Input: part model. Units: mm. Frame: model coordinates. Face numbers are marked on the shaded views. A direction names the side the tool comes from. Round coordinates to 2 decimals unless told otherwise and drop trailing zeros. Order: outer loops, then holes, each group sorted by start corner. A loop starts at its lowest first (then second) coordinate and runs counter-clockwise, first axis right, second up. Notation, with made-up numbers: (-9.75, 15.25) - (26.25, 15.25) arc R32 ccw to (26.25, 48.25) - close; hole circle Ø8 at (26, 26.25). An arc over 180 degrees is marked (long way). One line per item, written item: value. Start each with the question number.
Autodesk Inventor part; units mm, degrees
ref_plane "WorkPlane2" through (0, 0, 0) normal (0, 0, 1) x (1, 0, 0)
ref_plane "Work Plane2" through (0, 0, -2.35) normal (0, 0, 1) x (1, 0, 0)
ref_plane "WorkPlane3" through (0, 0, 7) normal (0, 0, 1) x (1, 0, 0)
ref_plane "WorkPlane2" through (0, 0, 0) normal (0, 0, 1) x (1, 0, 0)
sketch "Sketch1" plane through (0, 0, 0) normal (1, 0, 0) x (0, 1, 0)
  point P0 (0, 0)
ref_plane "Work Plane2" through (0, 0, -2.35) normal (0, 0, 1) x (1, 0, 0)
ref_plane "WorkPlane3" through (0, 0, 7) normal (0, 0, 1) x (1, 0, 0)
sketch "Sketch2" plane through (0, 0, 0) normal (0, 1, 0) x (-1, 0, 0)
  point P0 (0, 0)
sketch "Sketch3" plane through (0, 0, 0) normal (1, 0, 0) x (0, 1, 0)
  line L0 (1.5, -3.35) -> (1.25, -2.85)
  line L1 (1.5, -16.7) -> (1.5, -3.35)
  line L2 (0, -16.7) -> (1.5, -16.7)
  line L3 (0, 0) -> (0, -16.7)
  arc A0 (2.75, -0.7) -> (0, 0) centre (0, -5.7518) ccw
  line L4 (2.75, -0.85) -> (2.75, -0.7)
  line L5 (1.25, -2.35) -> (2.75, -0.85)
  line L6 (1.25, -2.85) -> (1.25, -2.35)
  line L7 (0, -31.6445) -> (0, 31.6445) construction
  line L8 (0, -31.6445) -> (0, 31.6445)
  line L9 (0, -44.3023) -> (0, 44.3023)
  dimension "d2" = 1.5
  dimension "d4" = 1.25
  dimension "d6" = 0.5
  dimension "d8" = 1.65
  dimension "d10" = 135
  dimension "d12" = 2.75
  dimension "d14" = 0
  dimension "d16" = 0.7
  dimension "d18" = 16
  dimension "d22" = 13.35
revolve "Revolution1" add sketch "Sketch3" angle 360 about axis through (0, 0, -31.6445) along (0, 0, 1)
fillet "Fillet1" radius 0.8 1 edges at (0, -1.25, -2.35)
sketch "Sketch4" plane through (0, 0, 0) normal (0, 1, 0) x (-1, 0, 0)
  line L0 (0, 0) -> (-1.7, 0)
  line L1 (0, -1.4167) -> (0, 0)
  line L2 (-1.7, 0) -> (-0.2833, -1.4167)
  line L3 (0, -6.9021) -> (0, 1.1504)
  arc A0 (2.75, -0.7) -> (-2.75, -0.7) centre (0, -5.7518) ccw
  line L4 (0, -1.4167) -> (-0.2833, -1.4167)
  point P0 (0, -1.7)
  dimension "d30" = 45
  dimension "d33" = 3.4
  dimension "d34" = 0.2833
  dimension "d35" = 90
extrude "Extrusion1" cut sketch "Sketch4" along normal mid plane 0.5667
pattern_circular "PolarArray1" count 4 over 360 about axis through (0, 0, -10) along (0, 0, 1) of "Extrusion1"
thread "Thread1"
ref_plane "MSC_PF1" through (0, 0, 0) normal (1, 0, 0) x (0, 1, 0)
ref_plane "MSC_PT1" through (0, 2.75, -0.85) normal (0, 0, -1) x (-1, 0, 0)
equation "\"d2\" = 0.5 * NND"
equation "\"d4\" = 0.5 * msp_mdtds"
equation "\"d6\" = msp_x"
equation "\"d8\" = ParK"
equation "\"d12\" = 0.5 * Dk"
equation "\"d16\" = ParF"
equation "\"d18\" = NLG"
equation "\"d22\" = b"
equation "\"d24\" = r"
equation "\"d33\" = M"
equation "\"d31\" = 0.166667 * M"
equation "\"d39\" = b"
equation "\"PTC\" = 0.5"
equation "\"msp_x\" = PTC"
equation "\"NLG\" = 16"
equation "\"NND\" = 3"
equation "\"ParK\" = 1.65"
equation "\"r\" = 0.8"
equation "\"msp_mdtds\" = NND - PTC"
equation "\"b\" = 13.35"
equation "\"Dk\" = 5.5"
equation "\"ParF\" = 0.7"
equation "\"M\" = 3.4"
equation "\"ParA\" = 1"
equation "\"THREADDIA\" = NND"
equation "\"TEMPLATE\" = 1.2345"
properties part number "ISO 7047 - M3x16 - 4.8 - H" material "Steel"
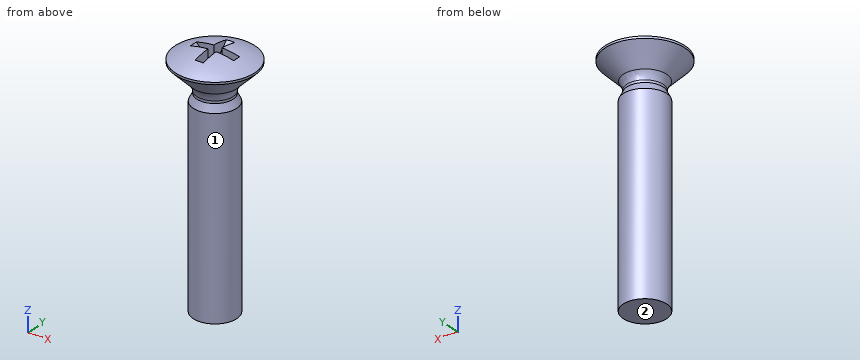
1. Pin query (flat end, axial travel): pin 1 (0.6 mm diameter, centred on x = 1, z = -0.5, fed in from +Y); pin 2 (1 mm diameter, centred on x = -1, z = -0.5, fed in from +Y); pin 3 (1.3 mm diameter, centred on y = -1, z = -1, fed in from -X). Return the tip coordinate at first contact, or that it passes through.
2. Line query: line 1 (Y direction, x = 0.15, z = -0.75); line 2 (X direction, y = -0.1, z = -5); line 3 (Z direction, x = -1.15, y = 0.9). Output: solid intervals per line, ascending. Write a range as from..to.
3. Section A-A (z = -1.25). Return the cut outline in (x, y).
4. Section B-B (z = -13). Return the cut outline in (x, y).
5. Set-up query: the marked faces 1 and 2. Return all of +Z, -Z, +X, -X, +Y, -Y with unobstructed straight access to the full face (end or side cutting, diameter ignored); none if empty.
Solved:
1. pin 1: stops at y = 2.64
1. pin 2: stops at y = 2.7
1. pin 3: stops at x = -2.73
2. line 1: y = -2.75..-0.95, 0.95..2.75
2. line 2: x = -1.5..1.5
2. line 3: z = -16.7..-3.27, -2.14..-0.19
3. outline: circle Ø4.7 at (0, 0); hole (-0.45, -0.28) - (-0.28, -0.28) - (-0.28, -0.45) - (0.28, -0.45) - (0.28, -0.28) - (0.45, -0.28) - (0.45, 0.28) - (0.28, 0.28) - (0.28, 0.45) - (-0.28, 0.45) - (-0.28, 0.28) - (-0.45, 0.28) - close
4. outline: circle Ø3 at (0, 0)
5. face 1: -Z
5. face 2: -Z, +X, -X, +Y, -Y
